```python
from build123d import *

# Parameters (mm, degrees)
SKETCH_1_W      = 60
SKETCH_1_H      = 60
EXTRUDE_1_DEPTH = 100
CHAMFER_1_SIZE  = 10
CHAMFER_2_SIZE  = 10
CHAMFER_3_SIZE  = 10
CHAMFER_4_SIZE  = 10
CHAMFER_5_SIZE  = 10
CHAMFER_6_SIZE  = 10
CHAMFER_7_SIZE  = 10
CHAMFER_8_SIZE  = 10
SKETCH_4_R      = 15
EXTRUDE_2_DEPTH = 3
SKETCH_5_R      = 4.130427407
EXTRUDE_3_DEPTH = 89
CHAMFER_9_SIZE  = 10
CHAMFER_10_SIZE = 10
CHAMFER_11_SIZE = 10


with BuildPart() as part:
    # 草图1 → 凸台-拉伸1 (new body)
    with BuildSketch(Plane.XY):
        Rectangle(SKETCH_1_W, SKETCH_1_H)
    extrude(amount=EXTRUDE_1_DEPTH)

    # 倒角1
    chamfer_1_edges = [part.edges().sort_by_distance(p)[0] for p in [
        (0, 30, 0),
    ]]
    chamfer(chamfer_1_edges, length=CHAMFER_1_SIZE)

    # 倒角2
    chamfer_2_edges = [part.edges().sort_by_distance(p)[0] for p in [
        (-30, -5, 0),
    ]]
    chamfer(chamfer_2_edges, length=CHAMFER_2_SIZE)

    # 倒角3
    chamfer_3_edges = [part.edges().sort_by_distance(p)[0] for p in [
        (5, -30, 0),
    ]]
    chamfer(chamfer_3_edges, length=CHAMFER_3_SIZE)

    # 倒角4
    chamfer_4_edges = [part.edges().sort_by_distance(p)[0] for p in [
        (30, 0, 0),
    ]]
    chamfer(chamfer_4_edges, length=CHAMFER_4_SIZE)

    # 倒角5
    chamfer_5_edges = [part.edges().sort_by_distance(p)[0] for p in [
        (0, 30, 100),
    ]]
    chamfer(chamfer_5_edges, length=CHAMFER_5_SIZE)

    # 倒角6
    chamfer_6_edges = [part.edges().sort_by_distance(p)[0] for p in [
        (30, -5, 100),
    ]]
    chamfer(chamfer_6_edges, length=CHAMFER_6_SIZE)

    # 倒角7
    chamfer_7_edges = [part.edges().sort_by_distance(p)[0] for p in [
        (-30, -5, 100),
    ]]
    chamfer(chamfer_7_edges, length=CHAMFER_7_SIZE)

    # 倒角8
    chamfer_8_edges = [part.edges().sort_by_distance(p)[0] for p in [
        (0, -30, 100),
    ]]
    chamfer(chamfer_8_edges, length=CHAMFER_8_SIZE)

    # 草图4 → 凸台-拉伸2 (add)
    with BuildSketch(Plane(origin=(0, 30, 0), x_dir=(1, 0, 0), z_dir=(0, 1, 0))):
        with Locations(Location((0, -50, 0), (0, 0, 90))):  # turned: the seam where the file's is
            Circle(SKETCH_4_R)
    extrude(amount=EXTRUDE_2_DEPTH)

    # 草图5 → 凸台-拉伸3 (add)
    with BuildSketch(Plane.XZ.offset(30)):
        with Locations(Location((0, 50, 0), (0, 0, 90))):  # turned: the seam where the file's is
            Circle(SKETCH_5_R)
    extrude(amount=EXTRUDE_3_DEPTH)

    # 倒角9
    chamfer_9_edges = [part.edges().sort_by_distance(p)[0] for p in [
        (30, 30, 50),
    ]]
    chamfer(chamfer_9_edges, length=CHAMFER_9_SIZE)

    # 倒角10
    chamfer_10_edges = [part.edges().sort_by_distance(p)[0] for p in [
        (-30, 30, 50),
    ]]
    chamfer(chamfer_10_edges, length=CHAMFER_10_SIZE)

    # 倒角11
    chamfer_11_edges = [part.edges().sort_by_distance(p)[0] for p in [
        (30, -30, 50),
    ]]
    chamfer(chamfer_11_edges, length=CHAMFER_11_SIZE)


solid = part.part
```
The model under review builds one solid part; all positions refer to its coordinate system, in mm. A direction names the side the tool comes from. Round coordinates to 2 decimals unless told otherwise and drop trailing zeros. Order: outer loops, then holes, each group sorted by start corner. A loop starts at its lowest first (then second) coordinate and runs counter-clockwise, first axis right, second up. Notation, with made-up numbers: M 2,-7.75 L 31,-7.75 A6 ccw 31,-2.75 Z; hole C 52,24.5 d4. An arc over 180 degrees is marked long. Use a Markdown table: item, result.
1) Consider section C-C (x = -23). Write out the cut boundary in (y, z), then the cut area to 3 significant figures.
Report:
| item | result |
|---|---|
| outline | M -30,10 L -23,3 L 23,3 L 27,7 L 27,93 L 23,97 L -23,97 L -30,90 Z |
| area | 5,290 mm^2 |
2) Consider section D-D (z = 30.5). Write out the cut boundary in (x, y).
Report:
| item | result |
|---|---|
| outline | M -30,-30 L 20,-30 L 30,-20 L 30,20 L 20,30 L -20,30 L -30,20 Z |
3) Consider section A-A (x = 12). Write out the cut boundary in (y, z), then the cut area to 3 significant figures.
Report:
| item | result |
|---|---|
| outline | M -30,10 L -20,0 L 20,0 L 30,10 L 30,41 L 33,41 L 33,59 L 30,59 L 30,90 L 20,100 L -20,100 L -30,90 Z |
| area | 5,850 mm^2 |
4) Wall thickness on line 1 along Y through (x, z) = (-8.5, 47); line 2 along Y through (x, z) = (-25, 30); line 3 along Z through (x, y) = (27.5, 20): over which ranges is each line inside the solid? List them lowest first. Write a range as [from, to].
Report:
| item | result |
|---|---|
| line 1 | [-30, 33] |
| line 2 | [-30, 25] |
| line 3 | [7.5, 92.5] |
5) Insertion check: pin 1 (8 mm diameter, centred on y = -91, z = 48.5, fed in from +X); pin 2 (1 mm diameter, centred on x = 2, y = -48, fed in from -Z); pin 3 (1 mm diameter, centred on x = -23.5, y = -19, fed in from -Z). Each pin has a flat end and moves straight along its axis. Give the tip position at first contact, or say it passes through.
Report:
| item | result |
|---|---|
| pin 1 | x = 4.13 |
| pin 2 | z = 46.15 |
| pin 3 | z = 3 |
6) Tool access review of faces 1 (the face through (25, -25, 49)), 2 (the face through (-0.66, 31.479, 64.985)), 3 (the face through (-0.182, -73.877, 45.874)): name each direction out of +Z, -Z, +X, -X, +Y, -Y from which nothing blocks a thin tool from reaching the whole face with its end or side.
Report:
| item | result |
|---|---|
| face 1 | +Z, -Z, +X, -Y |
| face 2 | +Y |
| face 3 | -Y |
7) Consider section B-B (z = 50). Write out the cut boundary in (x, y), then the cut area to 3 significant figures.
Report:
| item | result |
|---|---|
| outline | M -30,-30 L -4.13,-30 L -4.13,-119 L 4.13,-119 L 4.13,-30 L 20,-30 L 30,-20 L 30,20 L 20,30 L 15,30 L 15,33 L -15,33 L -15,30 L -20,30 L -30,20 Z |
| area | 4,280 mm^2 |
